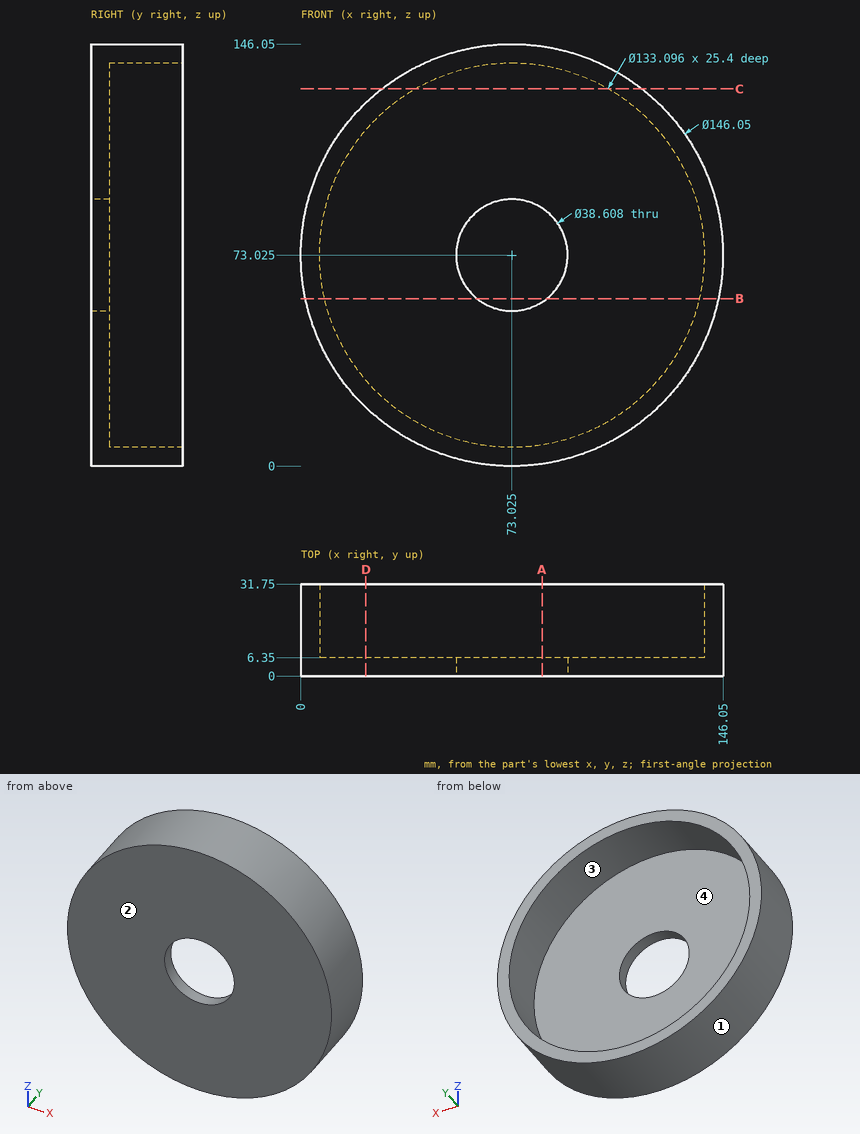
Verification items for this drawing (mm, ordinates from the low corner). Round coordinates to 2 decimals unless told otherwise and drop trailing zeros. Loops run counter-clockwise (first coordinate to the right, second up) from the corner with the lowest first, then second, coordinate; pieces in that order, holes last. Notation, with made-up numbers: (47.5, -11) -> (105.5, -11) arc R9 cw to (105.5, 3) -> close; hole circle Ø5 at (80, 83.5). An arc over 180 degrees is marked (long way). Write item = value, one per line. Start each with the question number.
1) Sectioned sample at C-C, the plane z = 130.5. Record the cut outline in (x, y).
2) Sectioned sample at A-A, the plane x = 83.5. Record the cut outline in (y, z).
3) Release check for a two-part mould opening along Z. For the marked faces 1, 2, 3 and 4 record: released by +Z, released by -Z, zero draft, split by the parting line, or undercut.
4) Sectioned sample at B-B, the plane z = 58. Record the cut outline in (x, y), plus the area to 3 significant figures.
5) Sectioned sample at D-D, the plane x = 22.5. Record the cut outline in (y, z).
6) Thickness scan on probe 1 along X at (y, z) = (8, 74.5); probe 2 along Z at (x, y) = (93, 24); probe 3 along Z at (x, y) = (103.5, 18.5). Record the ranges inside material, lowest first.
7) Gauge pin test, flat ends, axial feed: pin 1 Ø1 at (x, y) = (104, 10.5) entering from +Z; pin 2 Ø5 at (x, y) = (119.5, 24.5) entering from -Z; pin 3 Ø4 at (y, z) = (11.5, 26) entering from +X. Record the tip position at first contact, or that the pin passes through.
Results are:
q1.outline = (27.98, 0) -> (118.07, 0) -> (118.07, 31.75) -> (106.57, 31.75) -> (106.57, 6.35) -> (39.48, 6.35) -> (39.48, 31.75) -> (27.98, 31.75) -> close
q2.outline = (0, 0.76) -> (31.75, 0.76) -> (31.75, 7.31) -> (6.35, 7.31) -> (6.35, 56.81) -> (0, 56.81) -> close; (0, 89.24) -> (6.35, 89.24) -> (6.35, 138.74) -> (31.75, 138.74) -> (31.75, 145.29) -> (0, 145.29) -> close
q3.face_1 = split by the parting line
q3.face_2 = zero draft
q3.face_3 = undercut
q3.face_4 = undercut
q4.outline = (1.56, 0) -> (60.91, 0) -> (60.91, 6.35) -> (8.2, 6.35) -> (8.2, 31.75) -> (1.56, 31.75) -> close; (85.14, 0) -> (144.49, 0) -> (144.49, 31.75) -> (137.85, 31.75) -> (137.85, 6.35) -> (85.14, 6.35) -> close
q4.area = 1,090 mm^2
q5.outline = (0, 20.3) -> (31.75, 20.3) -> (31.75, 29.71) -> (6.35, 29.71) -> (6.35, 116.34) -> (31.75, 116.34) -> (31.75, 125.75) -> (0, 125.75) -> close
q6.probe_1 = 0.01 to 6.49, 139.56 to 146.04
q6.probe_2 = 2.79 to 9.55, 136.5 to 143.26
q6.probe_3 = 6.66 to 13.86, 132.19 to 139.39
q7.pin_1 = 139.39
q7.pin_2 = 14.73
q7.pin_3 = 130.52
